from build123d import *

# Parameters (mm, degrees)
SKETCH1_W           = 125
SKETCH1_H           = 80
BOSS_EXTRUDE1_DEPTH = 33
SKETCH3_W           = 120
SKETCH3_H           = 75
CUT_EXTRUDE1_DEPTH  = 30
SKETCH6_W           = 14.123986893
SKETCH6_H           = 14
SKETCH6_W_2         = 13.154693674
SKETCH6_H_2         = 11
CUT_EXTRUDE4_DEPTH  = 15
SKETCH7_W           = 6
SKETCH7_H           = 6.231170688
SKETCH7_W_2         = 18
CUT_EXTRUDE5_DEPTH  = 15


with BuildPart() as part:
    # Sketch1 → Boss-Extrude1 (new body)
    with BuildSketch(Plane(origin=(0, 0, 0), x_dir=(1, 0, 0), z_dir=(0, 1, 0))):
        with Locations((62.5, 40)):
            Rectangle(SKETCH1_W, SKETCH1_H)
    extrude(amount=BOSS_EXTRUDE1_DEPTH)

    # Sketch3 → Cut-Extrude1 (cut)
    with BuildSketch(Plane(origin=(0, 33, 0), x_dir=(1, 0, 0), z_dir=(0, 1, 0))):
        with Locations((62.403820475, 39.836034952)):
            Rectangle(SKETCH3_W, SKETCH3_H)
    extrude(amount=-CUT_EXTRUDE1_DEPTH, mode=Mode.SUBTRACT)

    # Sketch6 → Cut-Extrude4 (cut)
    with BuildSketch(Plane(origin=(0, 33, 0), x_dir=(1, 0, 0), z_dir=(0, 1, 0))):
        with Locations((0.880645417, 30)):
            Rectangle(SKETCH6_W, SKETCH6_H)
        with Locations((1.365292027, 44.5)):
            Rectangle(SKETCH6_W_2, SKETCH6_H_2)
    extrude(amount=-CUT_EXTRUDE4_DEPTH, mode=Mode.SUBTRACT)

    # Sketch7 → Cut-Extrude5 (cut)
    with BuildSketch(Plane(origin=(0, 0, -80), x_dir=(-1, 0, 0), z_dir=(0, 0, -1))):
        with Locations((-48, 16.115585344)):
            Rectangle(SKETCH7_W, SKETCH7_H)
        with Locations((-86, 16.115585344)):
            Rectangle(SKETCH7_W_2, SKETCH7_H)
    extrude(amount=-CUT_EXTRUDE5_DEPTH, mode=Mode.SUBTRACT)


solid = part.part
For this review, take the finished solid that the model builds, in its own axes (mm). A direction names the side the tool comes from. Round coordinates to 2 decimals unless told otherwise and drop trailing zeros. Write each loop counter-clockwise with the first axis right and the second up, starting at its lowest first coordinate (ties: lowest second). Pieces come first, ordered by that corner, then holes. Notation, with made-up numbers: (73.25, -19.75) - (87.25, -19.75) arc R18 ccw to (87.25, 7.25) - close; hole circle Ø1 at (75, -20). An arc over 180 degrees is marked (long way). Write item = value, one per line. Start each with the question number.
1. Consider section B-B on x = 88. State the section outline as (y, z) points.
2. For pin 1 Ø8 at (x, z) = (15.5, -33) entering from -Y; pin 2 Ø10 at (x, z) = (100, -28.5) entering from +Y; pin 3 Ø1.2 at (x, z) = (1, -33) entering from +Y, all flat-tipped, find the tip position at first contact; note any pin that passes through.
3. Consider section D-D on y = 10.5. State the section outline as (x, z) points, plus the area to 4 significant figures.
4. Consider section C-C on z = -33. State the section outline as (x, y) points, plus the area to 3 significant figures.
5. For faces 5 (the face through (62, 18, -77.336)), 6 (the face through (1, 18, -45)), 7 (the face through (48, 13, -79)), list the 3-axis set-ups (+Z, -Z, +X, -X, +Y, -Y) from which the entire face can be reached by the end or side of a thin tool; tool diameter is ignored.
6. Consider section A-A on y = 23.5. State the section outline as (x, z) points, plus the area to 3 significant figures.
7. Wall thickness on L1, parallel to Z at x = 73, y = 30; L2, parallel to X at y = 31.5, z = -4; L3, parallel to Y at x = 29, z = -75: over which ranges is each line inside the solid? List them lowest first.
8. Draft analysis for pull direction Y (two halves, no side actions). For faces 1 (the face through (62, 3, -40)), 2 (the face through (77, 16, -79)), 3 (the face through (86, 19.231, -79)), 4 (the face through (122.404, 18, -39)), state which applies: released by +Y, released by -Y, zero draft, split by the parting line, or undercut.
Evaluation:
q1.outline = (0, -80) - (13, -80) - (13, -77.34) - (3, -77.34) - (3, -2.34) - (33, -2.34) - (33, 0) - (0, 0) - close; (19.23, -80) - (33, -80) - (33, -77.34) - (19.23, -77.34) - close
q2.pin_1 = 0
q2.pin_2 = 3
q2.pin_3 = 18
q3.outline = (0, -80) - (125, -80) - (125, 0) - (0, 0) - close; hole (2.4, -77.34) - (122.4, -77.34) - (122.4, -2.34) - (2.4, -2.34) - close
q3.area = 1,000 mm2
q4.outline = (0, 0) - (125, 0) - (125, 33) - (122.4, 33) - (122.4, 3) - (2.4, 3) - (2.4, 18) - (0, 18) - close
q4.area = 489 mm2
q5.face_5 = +Y
q5.face_6 = -X, +Y
q5.face_7 = -Z
q6.outline = (0, -80) - (125, -80) - (125, 0) - (0, 0) - (0, -23) - (2.4, -23) - (2.4, -2.34) - (122.4, -2.34) - (122.4, -77.34) - (2.4, -77.34) - (2.4, -50) - (0, -50) - close; (0, -39) - (2.4, -39) - (2.4, -37) - (0, -37) - close
q6.area = 940 mm2
q7.L1 = -80 to -77.34, -2.34 to 0
q7.L2 = 0 to 2.4, 122.4 to 125
q7.L3 = 0 to 3
q8.face_1 = released by +Y
q8.face_2 = undercut
q8.face_3 = undercut
q8.face_4 = zero draft
